Autodesk Inventor part; units mm, degrees
ref_plane "YZ Plane" through (0, 0, 0) normal (1, 0, 0) x (0, 1, 0)
ref_plane "XZ Plane" through (0, 0, 0) normal (0, 1, 0) x (-1, 0, 0)
ref_plane "XY Plane" through (0, 0, 0) normal (0, 0, 1) x (1, 0, 0)
sketch "Sketch1" plane through (0, 0, 0) normal (0, 0, 1) x (1, 0, 0)
  circle A0 centre (0, 0) radius 1.5
  dimension "d0" = 3
extrude "Extrusion1" add sketch "Sketch1" along normal blind 10
sketch "Sketch2" plane through (0, 0, 0) normal (0, 0, -1) x (-1, 0, 0)
  circle A0 centre (0, 0) radius 1.5
  circle A1 centre (0, 0) radius 2.25
  dimension "d3" = 4.5
extrude "Extrusion2" add sketch "Sketch2" along normal blind 3 contours A0 | A1
sketch "Sketch3" plane through (0, 0, -3) normal (0, 0, -1) x (-1, 0, 0)
  circle A0 centre (0, 0) radius 2.25
  line L0 (-0.7217, 1.25) -> (0.7217, 1.25)
  line L1 (0.7217, 1.25) -> (1.4434, 0)
  line L2 (1.4434, 0) -> (0.7217, -1.25)
  line L3 (0.7217, -1.25) -> (-0.7217, -1.25)
  line L4 (-0.7217, -1.25) -> (-1.4434, 0)
  line L5 (-1.4434, 0) -> (-0.7217, 1.25)
  dimension "d6" = 2.5
extrude "Extrusion3" cut sketch "Sketch3" against normal blind 1.5 contours L0 L1 L2 L3 L4 L5
thread "Thread1"
chamfer "Chamfer1" distance 0.508 angle 45 1 edges at (-1.5, 0, 10)
chamfer "Chamfer2" distance 0.25 angle 45 1 edges at (2.25, 0, -3)
properties part number "m3 x10" material "Steel"
Model file for the job. Use its own axes, mm. A direction names the side the tool comes from. Coordinates: 2 decimals unless noted, no trailing zeros. Order: outer loops, then holes, each group sorted by start corner. A loop starts at its lowest first (then second) coordinate and runs counter-clockwise, first axis right, second up. Notation, with made-up numbers: (24.25, 64) -> (43.25, 64) arc R14 cw to (43.25, 85) -> close; hole circle Ø2 at (48.25, 76.25). An arc over 180 degrees is marked (long way). Return JSON: item names as keys, results as strings. Group by question number.
Item 1: Tool access for faces 1 (the flat face through (-1.08, 0.63, -2.26)), 2 (the cylindrical face through (-1.5, -0.07, 4.68)): list every direction of +Z, -Z, +X, -X, +Y, -Y with a clear straight run to the whole face (end or side of a thin tool).
Item 2: Wall check: line 1 along Y through (x, z) = (-0.1, 8); line 2 along Z through (x, y) = (-0.7, 0.1). Give the ranges that are in metal, low to high. Write a range as [from, to].
Item 3: Saw through at A-A on x = 0. Write the cut outline in (y, z), then the cut area to 3 significant figures.
Item 4: Saw through at B-B on z = 7.75. Write the cut outline in (x, y).
Item 5: Pull direction X, two halves, no side cores. Call faces 3 (the flat face through (-1.088, -0.616, -2.26)), 4 (the cylindrical face through (0.29, -2.23, -1.36)), 5 (the flat face through (0, 0, 10)): pulls with the +X half, pulls with the -X half, needs draft (parallel to the pull), parting line crosses it, or undercut.
Item 6: Flat gauge pins, fed straight in: P1, Ø1.5, axis at y = 1, z = 3, coming from the +X side; P2, Ø0.7, axis at x = 0.5, z = -2.5, coming from the +Y side (3 decimals). Where does each tip first touch, or does it go through?
Values found:
{
 "1": {"face 1": "-Z", "face 2": "+Z"},
 "2": {"line 1": "y = [-1.5, 1.5]", "line 2": "z = [-1.5, 10]"},
 "3": {"outline": "(-2.25, -2.75) -> (-2, -3) -> (-1.25, -3) -> (-1.25, -1.5) -> (1.25, -1.5) -> (1.25, -3) -> (2, -3) -> (2.25, -2.75) -> (2.25, 0) -> (1.5, 0) -> (1.5, 9.49) -> (0.99, 10) -> (-0.99, 10) -> (-1.5, 9.49) -> (-1.5, 0) -> (-2.25, 0) -> close", "area": "39.4 mm2"},
 "4": {"outline": "circle Ø3 at (0, 0)"},
 "5": {"face 3": "undercut", "face 4": "parting line crosses it", "face 5": "needs draft"},
 "6": {"P1": "stops at x = 1.48", "P2": "stops at y = 2.245"}
}
